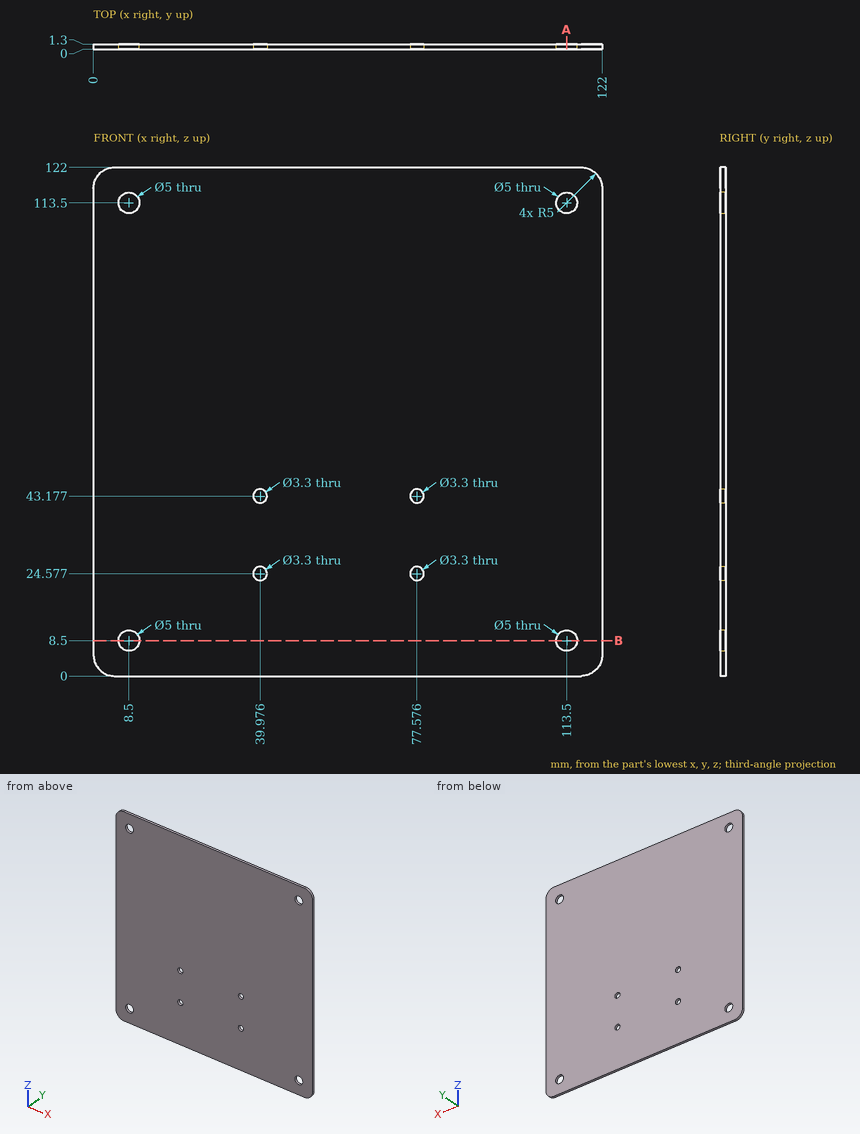
Study the drawing (mm; zero at the part's minimum x, y, z) and answer. Give positions to 0.01 mm unless a question says otherwise; leave off trailing zeros. Order: outer loops, then holes, each group sorted by start corner. A loop starts at its lowest first (then second) coordinate and runs counter-clockwise, first axis right, second up. Notation, with made-up numbers: (-35.75, 80.5) -> (-23.75, 80.5) arc R14 ccw to (-23.75, 95.5) -> close; hole circle Ø8 at (60.5, 76.25). An arc over 180 degrees is marked (long way). Write item = value, one per line.
1. A cutting plane is placed at B-B, the plane z = 8.5. Write down the section's boundary in (x, y).
Numbers:
outline = (0, 0) -> (6, 0) -> (6, 1.3) -> (0, 1.3) -> close; (11, 0) -> (111, 0) -> (111, 1.3) -> (11, 1.3) -> close; (116, 0) -> (122, 0) -> (122, 1.3) -> (116, 1.3) -> close
2. Given pin 1 (3 mm diameter, centred on x = 113.5, z = 8.5, fed in from -Y), flat-ended and moving along its own axis, determine where the tip first touches the part or whether it passes through.
Numbers:
pin_1 = through
3. A cutting plane is placed at A-A, the plane x = 113.5. Write down the section's boundary in (y, z).
Numbers:
outline = (0, 0) -> (1.3, 0) -> (1.3, 6) -> (0, 6) -> close; (0, 11) -> (1.3, 11) -> (1.3, 111) -> (0, 111) -> close; (0, 116) -> (1.3, 116) -> (1.3, 122) -> (0, 122) -> close
4. Straight lines are drawn through the part: line 1 along X through (y, z) = (0.25, 8.5); line 2 along X through (y, z) = (0.8, 43.5) (1 decimal). For each, find the intervals that lie inside material, in ascending order.
Numbers:
line_1 = 0 to 6, 11 to 111, 116 to 122
line_2 = 0 to 38.4, 41.6 to 76, 79.2 to 122
